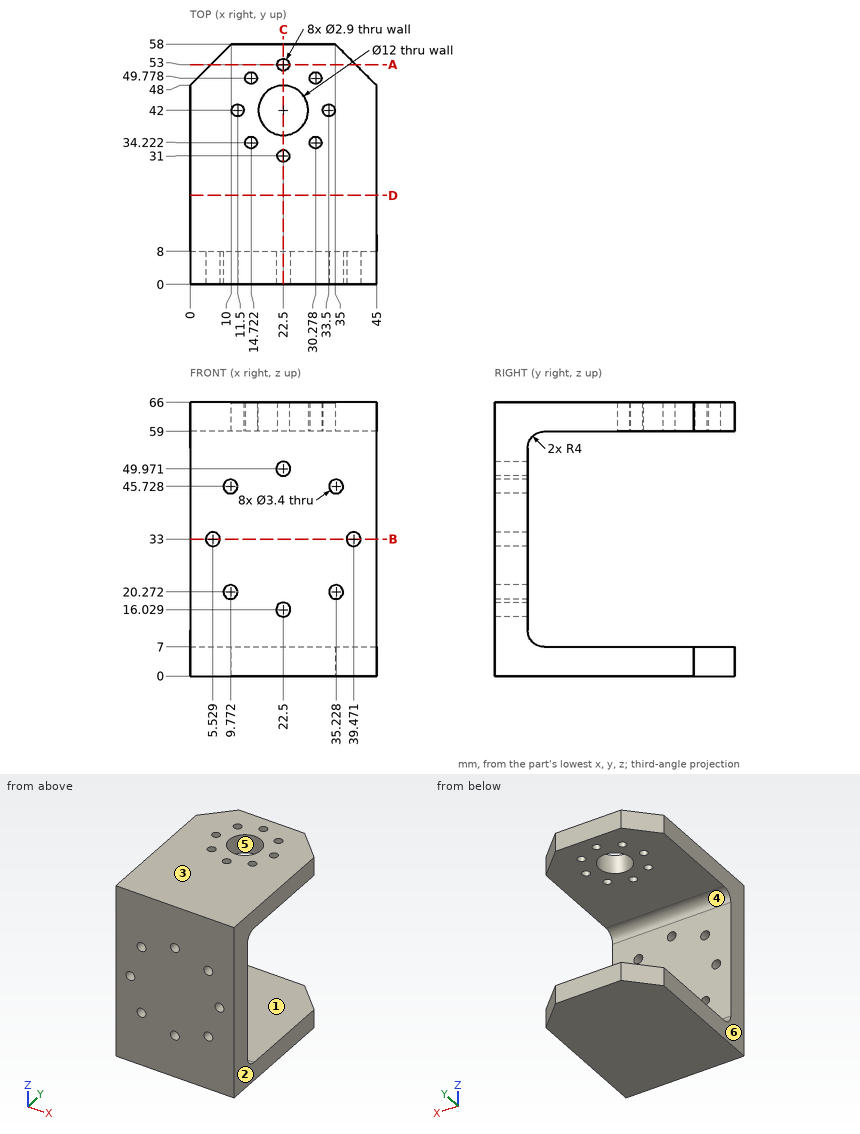
Job drawing, mm, ordinate dimensions from the low corner. One solid piece. A direction names the side the tool comes from. Round coordinates to 2 decimals unless told otherwise and drop trailing zeros. Loops run counter-clockwise (first coordinate to the right, second up) from the corner with the lowest first, then second, coordinate; pieces in that order, holes last.
Item 1: Cut at B-B, the plane z = 33. Give the cut face in (x, y).
Item 2: Cut at A-A, the plane y = 53. Give the cut face in (x, z).
Item 3: Drop flat-ended pins along their axis: P1, Ø5.5, axis at x = 22.5, z = 49.97, coming from the +Y side; P2, Ø2, axis at x = 35.23, z = 45.73, coming from the -Y side; P3, Ø2.5, axis at x = 33.5, y = 42, coming from the +Z side; P4, Ø6, axis at x = 5, z = 13, coming from the +Y side. Give the stop position or say it passes through.
Item 4: Drill centre lines: line 1 (Y direction, x = 22.5, z = 62.5); line 2 (Z direction, x = 23, y = 24); line 3 (Y direction, x = 6.5, z = 43). Where is each one in solid material? Low to high.
Item 5: 3-axis set-ups, long thin cutter, end or side, ignore diameter. For the marked faces 4, 5 and 6: which of +Z, -Z, +X, -X, +Y, -Y reach the whole face in a straight line?
Item 6: Cut at D-D, the plane y = 21.5. Give the cut face in (x, z).
Item 7: Cut at C-C, the plane x = 22.5. State how many separate pieces and enclosed holes the cut face has, then the cut area to 3 significant figures.
Item 8: Mould opens along Z. For the marked faces 1, 2 and 3 say: +Z half, -Z half, draft (parallel to the pull), parting line (faces both ways), or undercut.
A:
1. outline: (0, 0) - (3.83, 0) - (3.83, 8) - (0, 8) - close; (7.23, 0) - (37.77, 0) - (37.77, 8) - (7.23, 8) - close; (41.17, 0) - (45, 0) - (45, 8) - (41.17, 8) - close
2. outline: (5, 0) - (40, 0) - (40, 7) - (5, 7) - close; (5, 59) - (21.05, 59) - (21.05, 66) - (5, 66) - close; (23.95, 59) - (40, 59) - (40, 66) - (23.95, 66) - close
3. P1: stops at y = 8
3. P2: passes through
3. P3: stops at z = 7
3. P4: stops at y = 8.13
4. line 1: y = 0 to 29.55, 32.45 to 36, 48 to 51.55, 54.45 to 58
4. line 2: z = 0 to 7, 59 to 66
4. line 3: y = 0 to 8
5. face 4: +X, -X, +Y
5. face 5: +Z
5. face 6: +Z, -Z, -X, +Y, -Y
6. outline: (0, 0) - (45, 0) - (45, 7) - (0, 7) - close; (0, 59) - (45, 59) - (45, 66) - (0, 66) - close
7. separate pieces: 6
7. enclosed holes: 0
7. area: 1,060 mm2
8. face 1: undercut
8. face 2: draft
8. face 3: +Z half
